Autodesk Inventor part; units mm, degrees
ref_plane "YZ Plane" through (0, 0, 0) normal (1, 0, 0) x (0, 1, 0)
ref_plane "XZ Plane" through (0, 0, 0) normal (0, 1, 0) x (-1, 0, 0)
ref_plane "XY Plane" through (0, 0, 0) normal (0, 0, 1) x (1, 0, 0)
sketch "Sketch1" plane through (0, 0, 0) normal (0, 1, 0) x (-1, 0, 0)
  line L0 (21.75, 28.875) -> (-21.75, 28.875)
  line L1 (-21.75, 28.875) -> (-21.75, -28.875)
  line L2 (-21.75, -28.875) -> (21.75, -28.875)
  line L3 (21.75, -28.875) -> (21.75, 28.875)
  line L4 (21.75, 28.875) -> (-21.75, -28.875) construction
  line L5 (-21.75, 28.875) -> (21.75, -28.875) construction
  point P0 (0, 0)
  dimension "d0" = 43.5
  dimension "d1" = 57.75
extrude "Extrusion1" add sketch "Sketch1" along normal blind 6
fillet "Fillet1" radius 6 1 edges at (21.75, 6, 0)
fillet "Fillet2" radius 6 1 edges at (-21.75, 6, 0)
sketch "Sketch2" plane through (0, 0, 0) normal (0, -1, 0) x (1, 0, 0)
  line L0 (-21.75, 28.875) -> (21.75, 28.875)
  line L1 (-21.75, -28.875) -> (-21.75, 28.875)
  line L2 (21.75, -28.875) -> (-21.75, -28.875)
  line L3 (21.75, 28.875) -> (21.75, -28.875)
  line L4 (21.75, 28.875) -> (21.75, -28.875) construction
  line L5 (21.75, 28.875) -> (3.5, 28.875) construction
  line L6 (-21.75, 28.875) -> (21.75, 28.875) construction
  point P0 (0, 0)
  dimension "d6" = 18.25
extrude "Extrusion2" add sketch "Sketch2" along normal blind 8.5
sketch "Sketch3" plane through (-15.75, 6, 28.875) normal (0, 0, 1) x (1, 0, 0)
  arc A0 (0, 0) -> (-6, -6) centre (0, -6) ccw construction
  line L0 (-6, -6) -> (-6, -14.5) construction
  line L1 (37.5, -14.5) -> (-6, -14.5) construction
  line L2 (37.5, -6) -> (37.5, -14.5) construction
  arc A1 (37.5, -6) -> (31.5, 0) centre (31.5, -6) ccw construction
  line L3 (0, 0) -> (31.5, 0) construction
  line L4 (19.1951, -6) -> (19.1951, -10.25) construction
  point P0 (15.75, -6)
  dimension "d9" = 4.25
hole "Hole1" at (3.4451, -4.25, 28.875) direction (0, 0, -1) diameter 3.3 end through all
sketch "Sketch4" plane through (-15.75, 6, 28.875) normal (0, 0, 1) x (1, 0, 0)
  circle A0 centre (19.1951, -10.25) radius 1.65 construction
  line L0 (19.1951, -10.25) -> (19.1951, -14.5) construction
  line L1 (-6, -14.5) -> (37.5, -14.5) construction
  line L2 (37.5, -6) -> (37.5, -14.5)
  line L3 (19.1951, -14.5) -> (37.5, -6)
  line L4 (-6, -6) -> (-6, -14.5)
  line L5 (19.1951, -14.5) -> (-6, -6)
  line L6 (-6, -6) -> (-6, -14.5)
  line L7 (19.1951, -14.5) -> (37.5, -14.5)
  line L8 (37.5, -14.5) -> (37.5, -6)
  line L9 (19.1951, -14.5) -> (-6, -14.5)
  point P0 (15.75, -6)
extrude "Extrusion3" cut sketch "Sketch4" against normal through all
fillet "Fillet3" radius 6 1 edges at (3.4451, -8.5, 0)
ref_plane "Work Plane1" through (0, 0, 0) normal (0, 1, 0) x (1, 0, 0)
sketch "Sketch5" plane through (0, 0, 0) normal (0, 1, 0) x (1, 0, 0)
  line L0 (21.75, -28.875) -> (21.75, 28.875)
  line L1 (-21.75, 28.875) -> (-21.75, -28.875)
  line L2 (21.75, -23.875) -> (-21.75, -23.875)
  line L3 (-21.75, -23.875) -> (-21.75, 23.875)
  line L4 (-21.75, 23.875) -> (21.75, 23.875)
  line L5 (21.75, 23.875) -> (21.75, -23.875)
  line L6 (21.75, -28.875) -> (15.75, -28.875)
  line L7 (15.75, 28.875) -> (21.75, 28.875)
  point P0 (0, 0)
  dimension "d21" = 5
  dimension "d22" = 5
extrude "Extrusion4" cut sketch "Sketch5" against normal blind 8.5
sketch "Sketch6" plane through (0, 6, 0) normal (0, 1, 0) x (1, 0, 0)
  circle A0 centre (0, 0) radius 8
  dimension "d25" = 16
extrude "Extrusion5" cut sketch "Sketch6" against normal blind 8.5
sketch "Sketch7" plane through (0, 6, 0) normal (0, 1, 0) x (1, 0, 0)
  circle A0 centre (0, 0) radius 8
  circle A1 centre (0, 0) radius 13
  dimension "d28" = 5
extrude "Extrusion6" add sketch "Sketch7" along normal blind 10
fillet "Fillet4" radius 2 1 edges at (-13, 6, 0)
chamfer "Chamfer1" distance 3 angle 45 1 edges at (-8, 16, 0)
fillet "Fillet5" radius 2 2 edges at (-11, 16, 0) (-8, 13, 0)
fillet "Fillet6" radius 1 1 edges at (-13, 16, 0)
equation "\"d22\" = d21"
properties part number "support"
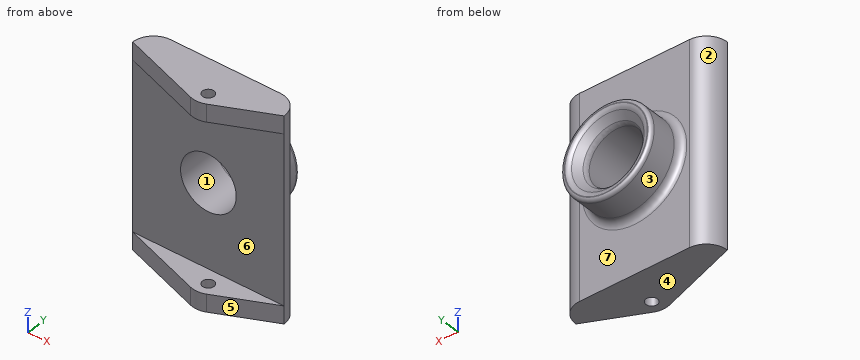
For this review, take the finished solid that the model builds, in its own axes (mm). Face numbers are marked on the shaded views. A direction names the side the tool comes from. Round coordinates to 2 decimals unless told otherwise and drop trailing zeros. Loops run counter-clockwise (first coordinate to the right, second up) from the corner with the lowest first, then second, coordinate; pieces in that order, holes last. Notation, with made-up numbers: (-7, -38.5) - (48, -38.5) arc R19 cw to (48, -25.5) - close; hole circle Ø6 at (39.5, 64). An arc over 180 degrees is marked (long way). One line per item, written item: value. Start each with the question number.
Item 1: The part is to be moulded in two halves that separate along Z. For the marked faces 1, 2, 3 and 4, say which applies: +Z half, -Z half, draft (parallel to the pull), parting line (faces both ways), or undercut.
Item 2: For the marked faces 5, 6 and 7, list the 3-axis set-ups (+Z, -Z, +X, -X, +Y, -Y) from which the entire face can be reached by the end or side of a thin tool; tool diameter is ignored.
Item 3: Clearance check with flat-ended pins moving along their axes: pin 1 Ø8 at (x, y) = (7, 10.5) entering from +Z; pin 2 Ø1 at (x, z) = (10, 12) entering from -Y; pin 3 Ø3 at (y, z) = (4.5, -2.5) entering from -X. State where each tip first meets the part, or that it passes through.
Item 4: Take a section at C-C (y = 2.75). Give the boundary of the cut face in (x, z) (3 decimals), plus the area to 3 significant figures.
Item 5: For L1, parallel to Z at x = 8.5, y = -1.25 (3 decimals); L2, parallel to X at y = 9, z = 0; L3, parallel to Y at x = -7.5, z = -14, list the stretches that pass through material, from the lowest coordinate up.
Item 6: Take a section at B-B (y = -4.25). Give the boundary of the cut face in (x, z) (3 decimals).
Answer below:
1. face 1: undercut
1. face 2: draft
1. face 3: parting line
1. face 4: -Z half
2. face 5: +Z, -Z, +X, -Y
2. face 6: +X, -X, -Y
2. face 7: +Y
3. pin 1: stops at z = 12.65
3. pin 2: stops at y = 0
3. pin 3: stops at x = -20.95
4. outline: (-21.083, -28.875) - (21.083, -28.875) - (21.083, 28.875) - (-21.083, 28.875) - close; hole circle Ø16 at (0, 0)
4. area: 2,230 mm2
5. L1: z = -28.875 to -23.875, 23.875 to 28.875
5. L2: x = -13 to -8, 8 to 13
5. L3: y = 0 to 6
6. outline: (-9.152, -28.875) - (1.795, -28.875) - (1.795, -23.875) - (-9.152, -23.875) - close; (-9.152, 23.875) - (1.795, 23.875) - (1.795, 28.875) - (-9.152, 28.875) - close; (5.095, -28.875) - (12.598, -28.875) - (12.598, -23.875) - (5.095, -23.875) - close; (5.095, 23.875) - (12.598, 23.875) - (12.598, 28.875) - (5.095, 28.875) - close
